The model under review builds one solid part; all positions refer to its coordinate system, in mm. Give positions to 0.01 mm unless a question says otherwise; leave off trailing zeros. Order: outer loops, then holes, each group sorted by start corner. A loop starts at its lowest first (then second) coordinate and runs counter-clockwise, first axis right, second up.
```python
from build123d import *

# Parameters (mm, degrees)
SKETCH_1_W      = 38
SKETCH_1_H      = 16
EXTRUDE_1_DEPTH = 7.2
SKETCH_2_R      = 0.25
EXTRUDE_2_DEPTH = 6.3


with BuildPart() as part:
    # 草图1 → 拉伸1 (new body)
    with BuildSketch(Plane(origin=(0, 0, 0), x_dir=(1, 0, 0), z_dir=(0, 1, 0))):
        Rectangle(SKETCH_1_W, SKETCH_1_H)
    extrude(amount=EXTRUDE_1_DEPTH)

    # 草图2 → 拉伸2 (add)
    with BuildSketch(Plane.XZ):
        with Locations(Location((6.224686657, 4.1, 0), (0, 0, 90))):
            Circle(SKETCH_2_R)
        with Locations(Location((3.734811994, 4.1, 0), (0, 0, 90))):
            Circle(SKETCH_2_R)
        with Locations(Location((1.244937331, 4.1, 0), (0, 0, 90))):
            Circle(SKETCH_2_R)
        with Locations(Location((-1.244937331, 4.1, 0), (0, 0, 90))):
            Circle(SKETCH_2_R)
        with Locations(Location((-3.734811994, 4.1, 0), (0, 0, 90))):
            Circle(SKETCH_2_R)
        with Locations(Location((-6.224686657, 4.1, 0), (0, 0, 90))):
            Circle(SKETCH_2_R)
        with Locations(Location((-6.224686657, -4.1, 0), (0, 0, 90))):
            Circle(SKETCH_2_R)
        with Locations(Location((-3.734811994, -4.1, 0), (0, 0, 90))):
            Circle(SKETCH_2_R)
        with Locations(Location((-1.244937331, -4.1, 0), (0, 0, 90))):
            Circle(SKETCH_2_R)
        with Locations(Location((1.244937331, -4.1, 0), (0, 0, 90))):
            Circle(SKETCH_2_R)
        with Locations(Location((3.734811994, -4.1, 0), (0, 0, 90))):
            Circle(SKETCH_2_R)
        with Locations(Location((6.224686657, -4.1, 0), (0, 0, 90))):
            Circle(SKETCH_2_R)
    extrude(amount=EXTRUDE_2_DEPTH)


solid = part.part
```
1. Take a section at A-A (y = -4.5). Count the separate pieces of the cut face and the enclosed holes in it, and give its area (3 significant figures).
2. Take a section at B-B (x = -7). Write out the cut boundary in (y, z), and give its area (3 significant figures).
3. To check wall thickness, follow line 1 (Y direction, x = -15.5, z = 0.5). State the ranges of the line that lie inside material, in increasing order.
4. Take a section at C-C (z = 5.5). Write out the cut boundary in (x, y), and give its area (3 significant figures).
Answer:
1. separate pieces: 12
1. enclosed holes: 0
1. area: 2.36 mm2
2. outline: (0, -8) - (7.2, -8) - (7.2, 8) - (0, 8) - close
2. area: 115 mm2
3. line 1: y = 0 to 7.2
4. outline: (-19, 0) - (19, 0) - (19, 7.2) - (-19, 7.2) - close
4. area: 274 mm2
